Geometry: final body of the model. Coordinates: model frame, mm. A direction names the side the tool comes from. Give positions to 0.01 mm unless a question says otherwise; leave off trailing zeros. Loops run counter-clockwise (first coordinate to the right, second up) from the corner with the lowest first, then second, coordinate; pieces in that order, holes last.
1. First-contact query: P1, Ø6, axis at x = 33.5, z = 24.5, coming from the +Y side; P2, Ø10, axis at x = -10.5, y = 76, coming from the +Z side; P3, Ø6, axis at x = 5.5, y = 24, coming from the +Z side. Flat tips, straight axial feed; report the tip coordinate or a pass-through.
2. Draft query along Y for faces 1 (the face through (6, 64.4, 14)), 2 (the face through (-19.524, 35.991, -4.336)), 3 (the face through (38.7, 7.2, -0.8)). Return one class per face: +Y half, -Y half, draft (parallel to the pull), parting line (faces both ways), or undercut.
3. Section A-A, the plane x = 0. State how many separate pieces and enclosed holes the cut face has, then the cut area to 3 significant figures.
4. Section D-D, the plane z = -32.5. Output: boundary loops of the cut face in (x, y), then the cut area to 3 significant figures.
5. Section C-C, the plane y = 6. Output: boundary loops of the cut face in (x, z).
6. Access query for faces 4 (the face through (-19, 0, -1)), 5 (the face through (-11.56, 76.57, -15.08)), 6 (the face through (17, 58.4, -11)). Directions: +Z, -Z, +X, -X, +Y, -Y. A direction counts if a zero-diameter tool reaches every point of the face in a straight line with its end or side. Return the directions, or none.
7. Material intervals for line 1 along X through (y, z) = (10.25, 0); line 2 along Y through (x, z) = (-16, 16); line 3 along X through (y, z) = (27, 0), sorted ascending.
from build123d import *

# Parameters (mm, degrees)
CROQUIS2_R              = 45
SALIENTE_EXTRUIR1_DEPTH = 14.2
CROQUIS3_R              = 20
SALIENTE_EXTRUIR3_DEPTH = 77.4
CROQUIS7_R              = 25
SALIENTE_EXTRUIR5_DEPTH = 30
CROQUIS13_R             = 15
CORTAR_EXTRUIR4_DEPTH   = 64.4
CHAFL_N1_SIZE           = 3
CHAFL_N1_SIZE2          = 3.5
CROQUIS14_R             = 19
CORTAR_EXTRUIR5_DEPTH   = 24
CROQUIS15_R             = 6.25
CORTAR_EXTRUIR6_DEPTH   = 14.2


with BuildPart() as part:
    # Croquis2 → Saliente-Extruir1 (new body)
    with BuildSketch(Plane(origin=(0, 0, 0), x_dir=(1, 0, 0), z_dir=(0, 1, 0))):
        with Locations(Location((0, 0, 0), (0, 0, 270))):
            Circle(CROQUIS2_R)
    extrude(amount=SALIENTE_EXTRUIR1_DEPTH)

    # Croquis3 → Saliente-Extruir3 (add)
    with BuildSketch(Plane(origin=(0, 0, 0), x_dir=(1, 0, 0), z_dir=(0, 1, 0))):
        with Locations(Location((0, 0, 0), (0, 0, 270))):
            Circle(CROQUIS3_R)
    extrude(amount=SALIENTE_EXTRUIR3_DEPTH)

    # Croquis7 → Saliente-Extruir5 (add)
    with BuildSketch(Plane(origin=(0, 58.4, 0), x_dir=(1, 0, 0), z_dir=(0, 1, 0))):
        with Locations(Location((0, 0, 0), (0, 0, 270))):
            Circle(CROQUIS7_R)
    extrude(amount=SALIENTE_EXTRUIR5_DEPTH)

    # Croquis13 → Cortar-Extruir4 (cut)
    with BuildSketch(Plane(origin=(0, 0, 0), x_dir=(1, 0, 0), z_dir=(0, 1, 0))):
        with Locations(Location((0, 0, 0), (0, 0, 270))):
            Circle(CROQUIS13_R)
    extrude(amount=CORTAR_EXTRUIR4_DEPTH, mode=Mode.SUBTRACT)

    # Chaflán1
    chafl_n1_edges = [part.edges().sort_by_distance(p)[0] for p in [
        (0, 0, -15),
    ]]
    chafl_n1_side = [part.faces().sort_by_distance(p)[0] for p in [
        (0, 32.2, -15),
    ]]
    chamfer(chafl_n1_edges, length=CHAFL_N1_SIZE, length2=CHAFL_N1_SIZE2, reference=chafl_n1_side[0])

    # Croquis14 → Cortar-Extruir5 (cut)
    with BuildSketch(Plane(origin=(0, 88.4, 0), x_dir=(1, 0, 0), z_dir=(0, 1, 0))):
        with Locations(Location((0, 0, 0), (0, 0, 270))):
            Circle(CROQUIS14_R)
    extrude(amount=-CORTAR_EXTRUIR5_DEPTH, mode=Mode.SUBTRACT)

    # Croquis15 → Cortar-Extruir6 (cut)
    with BuildSketch(Plane(origin=(0, 14.2, 0), x_dir=(1, 0, 0), z_dir=(0, 1, 0))):
        with Locations(Location((0, -32.5, 0), (0, 0, 270))):
            Circle(CROQUIS15_R)
        with Locations(Location((-32.5, 0, 0), (0, 0, 270))):
            Circle(CROQUIS15_R)
        with Locations(Location((0, 32.5, 0), (0, 0, 270))):
            Circle(CROQUIS15_R)
        with Locations(Location((32.5, 0, 0), (0, 0, 270))):
            Circle(CROQUIS15_R)
    extrude(amount=-CORTAR_EXTRUIR6_DEPTH, mode=Mode.SUBTRACT)


solid = part.part
Answers below:
1. P1: stops at y = 14.2
1. P2: stops at z = 24.39
1. P3: stops at z = 19.84
2. face 1: +Y half
2. face 2: undercut
2. face 3: draft
3. separate pieces: 4
3. enclosed holes: 0
3. area: 1,340 mm2
4. outline: (-31.12, 0) - (-6.25, 0) - (-6.25, 14.2) - (-31.12, 14.2) - close; (6.25, 0) - (31.12, 0) - (31.12, 14.2) - (6.25, 14.2) - close
4. area: 706 mm2
5. outline: circle Ø90 at (0, 0); hole circle Ø12.5 at (-32.5, 0); hole circle Ø30 at (0, 0); hole circle Ø12.5 at (0, -32.5); hole circle Ø12.5 at (0, 32.5); hole circle Ø12.5 at (32.5, 0)
6. face 4: +Z, -Z, +X, -X, -Y
6. face 5: +Y
6. face 6: none
7. line 1: x = -45 to -38.75, -26.25 to -15, 15 to 26.25, 38.75 to 45
7. line 2: y = 0 to 14.2, 58.4 to 88.4
7. line 3: x = -20 to -15, 15 to 20
